Could you check a few things on this model? Use its own coordinates, in mm. Face numbers are marked on the shaded views. A direction names the side the tool comes from. Coordinates: 2 decimals unless noted, no trailing zeros. Loops run counter-clockwise (first coordinate to the right, second up) from the corner with the lowest first, then second, coordinate; pieces in that order, holes last. Notation, with made-up numbers: (53.25, 86) - (94.25, 86) arc R28 cw to (94.25, 108) - close; hole circle Ø8 at (37.5, 83). An arc over 180 degrees is marked (long way). One line per question, with ' | ' between items. Start each with the question number.
1. We'd pull the mould along Z, two halves only. Please class the marked faces 1, 2 and 3: pulls with the +Z half, pulls with the -Z half, needs draft (parallel to the pull), parting line crosses it, or undercut.
2. I want a section at B-B, the plane y = 0. Write out the boundary of the cut face in (x, z), then the cut area to 3 significant figures.
3. Please list where these lines run through material, in increasing order: L1, parallel to Z at x = -67.5, y = 9; L2, parallel to Y at x = -63.5, z = 48.5; L3, parallel to X at y = -16.5, z = 27.5. Write a range as [from, to].
4. Which directions (+Z, -Z, +X, -X, +Y, -Y) give clear straight access to the entire face, cutting with the end or side of a thin tool? Please do the marked faces 4 and 5.
5. I want a section at C-C, the plane z = 39. Write out the boundary of the cut face in (x, y).
6. I'm going to push flat-ended pins straight in: P1, Ø1, axis at x = -47.5, y = 32, coming from the -Z side; P2, Ø20, axis at y = -4.5, z = 34, coming from the -X side. Where does each tip first touch, or does it pass through?
7. I want a section at D-D, the plane x = -39. Write out the boundary of the cut face in (y, z), then the cut area to 3 significant figures.
8. I want a section at A-A, the plane x = 58.64. Write out the boundary of the cut face in (y, z).
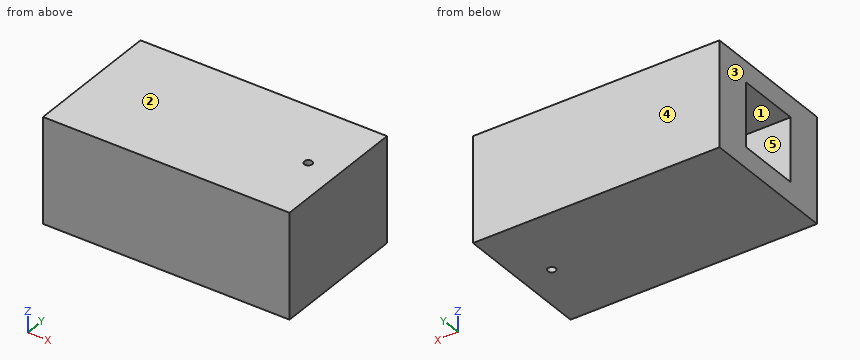
from build123d import *

# Parameters (mm, degrees)
IZIM1_W                     = 155
IZIM1_H                     = 87.2
Y_KSEKLIK_EKSTR_ZYON1_DEPTH = 66
IZIM2_R                     = 2.5
KES_EKSTR_ZYON1_DEPTH       = 111.739378723
IZIM3_W                     = 40
IZIM3_H                     = 40
KES_EKSTR_ZYON2_DEPTH       = 112


with BuildPart() as part:
    # Çizim1 → Yükseklik-Ekstrüzyon1 (new body)
    with BuildSketch(Plane.XY):
        Rectangle(IZIM1_W, IZIM1_H)
    extrude(amount=Y_KSEKLIK_EKSTR_ZYON1_DEPTH)

    # Çizim2 → Kes-Ekstrüzyon1 (cut, through all)
    with BuildSketch(Plane.XY.offset(66)):
        with Locations((58.64, 0)):
            Circle(IZIM2_R)
    extrude(amount=-KES_EKSTR_ZYON1_DEPTH, mode=Mode.SUBTRACT)

    # Çizim3 → Kes-Ekstrüzyon2 (cut)
    with BuildSketch(Plane.ZY.offset(77.5)):
        with Locations((33, 0)):
            Rectangle(IZIM3_W, IZIM3_H)
    extrude(amount=-KES_EKSTR_ZYON2_DEPTH, mode=Mode.SUBTRACT)


solid = part.part
Results are:
1) face 1: undercut | face 2: pulls with the +Z half | face 3: needs draft
2) outline: (-77.5, 0) - (56.14, 0) - (56.14, 66) - (-77.5, 66) - (-77.5, 53) - (34.5, 53) - (34.5, 13) - (-77.5, 13) - close; (61.14, 0) - (77.5, 0) - (77.5, 66) - (61.14, 66) - close | area: 5,420 mm2
3) L1: z = [0, 13], [53, 66] | L2: y = [-43.6, -20], [20, 43.6] | L3: x = [34.5, 77.5]
4) face 4: +Z, -Z, +X, -X, +Y | face 5: -X
5) outline: (-77.5, -43.6) - (77.5, -43.6) - (77.5, 43.6) - (-77.5, 43.6) - (-77.5, 20) - (34.5, 20) - (34.5, -20) - (-77.5, -20) - close; hole circle Ø5 at (58.64, 0)
6) P1: stops at z = 0 | P2: stops at x = 34.5
7) outline: (-43.6, 0) - (43.6, 0) - (43.6, 66) - (-43.6, 66) - close; hole (-20, 13) - (20, 13) - (20, 53) - (-20, 53) - close | area: 4,160 mm2
8) outline: (-43.6, 0) - (-2.5, 0) - (-2.5, 66) - (-43.6, 66) - close; (2.5, 0) - (43.6, 0) - (43.6, 66) - (2.5, 66) - close
